Autodesk Inventor part; units mm, degrees
ref_plane "YZ Plane" through (0, 0, 0) normal (1, 0, 0) x (0, 1, 0)
ref_plane "XZ Plane" through (0, 0, 0) normal (0, 1, 0) x (-1, 0, 0)
ref_plane "XY Plane" through (0, 0, 0) normal (0, 0, 1) x (1, 0, 0)
sketch "Sketch1" plane through (0, 0, 0) normal (0, 0, 1) x (1, 0, 0)
  line L0 (-45, 10) -> (45, 10)
  line L1 (45, 10) -> (45, -10)
  line L2 (45, -10) -> (-45, -10)
  line L3 (-45, -10) -> (-45, 10)
  line L4 (0, 0) -> (0, 7.2508) construction
  line L5 (0, 0) -> (8.0596, 0) construction
  dimension "d0" = 90
  dimension "d1" = 20
extrude "Plate1" add sketch "Sketch1" along normal blind 1.5
fillet "Fillet1" radius 2 4 edges at (45, 10, 0.75) (45, -10, 0.75) (-45, -10, 0.75) (-45, 10, 0.75)
sketch "Sketch2" plane through (0, 0, 1.5) normal (0, 0, 1) x (1, 0, 0)
  line L0 (-45, -8) -> (-45, 8)
  line L1 (45, 8) -> (45, -8)
  arc A0 (32.65, 0) -> (36.85, 0) centre (34.75, 0) ccw
  line L2 (36.85, 0) -> (36.85, 10)
  line L3 (32.65, 0) -> (32.65, 10)
  line L4 (43, -10) -> (-43, -10)
  line L5 (-43, 10) -> (43, 10)
  point P0 (0, 0)
  dimension "d5" = 10.25
  dimension "d6" = 4.2
  dimension "d7" = 10
extrude "Cut1" cut sketch "Sketch2" against normal blind 1.5
sketch "Sketch3" plane through (0, 0, 1.5) normal (0, 0, 1) x (1, 0, 0)
  line L0 (-45, -8) -> (-45, 8)
  point P0 (0, 0)
  point P1 (-34.75, 0)
  dimension "d10" = 10.25
hole "Hole1" at (-34.75, 0, 1.5) direction (0, 0, -1) diameter 4.2 depth 1.5 tip angle 118
sketch "Sketch5" plane through (0, 0, 1.5) normal (0, 0, 1) x (1, 0, 0)
  circle A0 centre (34.0345, 9.9478) radius 2.121
  arc A1 (32.65, 0) -> (36.85, 0) centre (34.75, 0) ccw
  line L0 (34.75, 0) -> (34.0345, 9.9478)
  line L1 (32.65, 0) -> (31.9141, 10)
  line L2 (-43, 10) -> (32.65, 10)
  line L3 (36.85, 0) -> (36.1504, 10.0945)
  line L4 (32.65, 0) -> (32.65, 10)
  line L5 (32.65, 0) -> (32.65, 10)
  line L6 (32.65, 10) -> (31.9141, 10)
  line L7 (32.65, 10) -> (32.65, 0)
  line L8 (32.65, 0) -> (31.35, 10)
  line L9 (-43, 10) -> (32.65, 10)
  line L10 (31.35, 10) -> (32.65, 10)
  point P0 (0, 0)
  dimension "d20" = 1.3
extrude "Cut2" cut sketch "Sketch5" against normal blind 1.5 contours L1 A0 | L2 L4 A0 L1 | A0 L1 L8 L2 | L4 L1 A0
equation "\"d8\" = Thickness"
equation "\"d16\" = Thickness"
equation "\"d18\" = Thickness"
equation "\"d2\" = Thickness"
equation "\"BendRadius\" = Thickness"
equation "\"BendReliefWidth\" = Thickness"
equation "\"BendReliefDepth\" = 0.5 * Thickness"
equation "\"CornerReliefSize\" = 4 * Thickness"
equation "\"MinimumRemnant\" = 2 * Thickness"
equation "\"TransitionRadius\" = BendRadius"
equation "\"JacobiRadiusSize\" = BendRadius"
equation "\"GapSize\" = Thickness"
properties part number "3d_LM-Welding_Tooling -  Tab" material "Aluminium 6061-T6"
The listing builds one solid part. Answer for the finished solid, in the listing's coordinates (mm). A direction names the side the tool comes from. Round coordinates to 2 decimals unless told otherwise and drop trailing zeros. Loops run counter-clockwise (first coordinate to the right, second up) from the corner with the lowest first, then second, coordinate; pieces in that order, holes last.
Q1. Section A-A, the plane y = 6 is taken. Determine the outline of the cut face in (x, z).
Q2. For a pull along X with two mould halves and no side action, classify faces 1 (the face through (44.43, 9.4, 0.76)), 2 (the face through (36.85, 5, 1)), 3 (the face through (-1, 0, 0)) as released by +X, released by -X, zero draft, split by the parting line, or undercut.
Q3. Section B-B, the plane x = -34.75 is taken. Determine the outline of the cut face in (y, z).
Q4. Find the intervals of material crossed by line 1 (X direction, y = 0, z = 1.1); line 2 (Y direction, x = -34.75, z = 0.95); line 3 (X direction, y = -0.5, z = 1.1), in increasing order.
Q5. Which of the six approach directions +Z, -Z, +X, -X, +Y, -Y give full straight-line access (tool end or side, diameter ignored) to faces 4 (the face through (32, 5, 1)), 5 (the face through (-32.7, 0.46, 0.74))?
Q6. Section C-C, the plane z = 0.45 is taken. Determine the outline of the cut face in (x, y), then the cut area to 3 significant figures.
Completed:
1. outline: (-45, 0) - (31.87, 0) - (31.87, 1.5) - (-45, 1.5) - close; (36.85, 0) - (45, 0) - (45, 1.5) - (36.85, 1.5) - close
2. face 1: released by +X
2. face 2: undercut
2. face 3: zero draft
3. outline: (-10, 0) - (-2.1, 0) - (-2.1, 1.5) - (-10, 1.5) - close; (2.1, 0) - (10, 0) - (10, 1.5) - (2.1, 1.5) - close
4. line 1: x = -45 to -36.85, -32.65 to 32.65, 36.85 to 45
4. line 2: y = -10 to -2.1, 2.1 to 10
4. line 3: x = -45 to -36.79, -32.71 to 32.71, 36.79 to 45
5. face 4: +Z, -Z, +Y
5. face 5: +Z, -Z
6. outline: (-45, -8) arc R2 ccw to (-43, -10) - (43, -10) arc R2 ccw to (45, -8) - (45, 8) arc R2 ccw to (43, 10) - (36.85, 10) - (36.85, 0) arc R2.1 cw to (32.65, 0) - (31.35, 10) - (-43, 10) arc R2 ccw to (-45, 8) - close; hole circle Ø4.2 at (-34.75, 0)
6. area: 1,730 mm2
